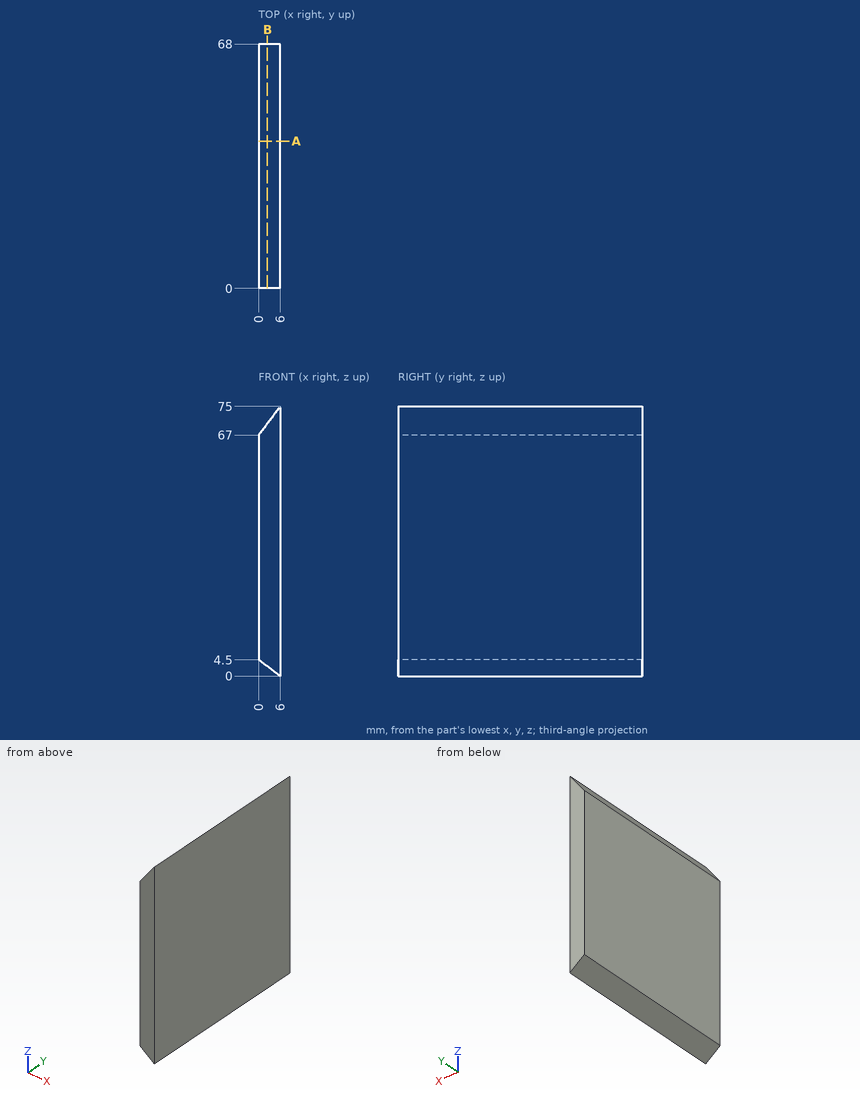
Study the drawing (mm; zero at the part's minimum x, y, z) and answer. Coordinates: 2 decimals unless noted, no trailing zeros. Order: outer loops, then holes, each group sorted by start corner. A loop starts at its lowest first (then second) coordinate and runs counter-clockwise, first axis right, second up. Notation, with made-up numbers: (29, -8.75) -> (78, -8.75) arc R30 cw to (78, 19.25) -> close; hole circle Ø10 at (-35.5, -5). An arc over 180 degrees is marked (long way). Answer in a Markdown table with one row per item. Add a question column.
Item 1: Find section B-B (x = 2.5). Write down the section's boundary in (y, z) (3 decimals), then the cut area to 3 significant figures.
Item 2: Find the intervals of material crossed by L1, parallel to Z at x = 2.5, y = 7.5 (3 decimals); L2, parallel to Z at x = 5.5, y = 28 (3 decimals); L3, parallel to X at y = 56, z = 70, in increasing order. Write a range as from..to.
Item 3: Find section A-A (y = 41). Write down the section's boundary in (x, z).
Item 4: This flat-tipped pin is pushed along its axis until it touches: P1, Ø2, axis at x = 1.5, y = 31.5, coming from the +Z side. Where does it stop, or does it pass through?
Result set:
| question | item | result |
|---|---|---|
| 1 | outline | (0, 2.625) -> (68, 2.625) -> (68, 70.333) -> (0, 70.333) -> close |
| 1 | area | 4,600 mm² |
| 2 | L1 | z = 2.625..70.333 |
| 2 | L2 | z = 0.375..74.333 |
| 2 | L3 | x = 2.25..6 |
| 3 | outline | (0, 4.5) -> (6, 0) -> (6, 75) -> (0, 67) -> close |
| 4 | P1 | stops at z = 70.33 |
